Work out the finished part from the listing and answer in its coordinate system (mm). A direction names the side the tool comes from. Give positions to 0.01 mm unless a question says otherwise; leave off trailing zeros. Write each loop counter-clockwise with the first axis right and the second up, starting at its lowest first coordinate (ties: lowest second). Pieces come first, ordered by that corner, then holes.
1) Determine the mould class of faces 1 (the face through (20, 20, -8)), 2 (the face through (-28.977, 29.58, -1.162)), 3 (the face through (3.228, 51.208, -0.406)), 4 (the face through (20, 20, 8)) for opening direction Z: pulls with the +Z half, pulls with the -Z half, needs draft (parallel to the pull), parting line crosses it, or undercut.
2) Find section C-C (x = -15). Determine the outline of the cut face in (y, z).
3) Find section A-A (z = 0). Determine the outline of the cut face in (x, y).
4) Find section B-B (y = 41.5). Determine the outline of the cut face in (x, z), plus the area to 3 significant figures.
5) Given pin 1 Ø2 at (x, y) = (-17.5, 9.5) entering from +Z; pin 2 Ø14 at (x, y) = (21, 17) entering from -Z; pin 3 Ø13 at (y, z) = (26.5, -4) entering from +X, each flat-ended and moving along its own axis, determine where each tip first touches the part or whether it passes through.
6) A tool of negligible diameter and unlimited length cuts with its end or side. For faces 5 (the face through (15.144, 22, 0)), 6 (the face through (-1, 0, 0)), from which of +Z, -Z, +X, -X, +Y, -Y can it reach the whole face along a straight path? Write none if from no direction.
7) Find section D-D (z = -14.5). Determine the outline of the cut face in (x, y).
8) Straight lines are drawn through the part: probe 1 along Z at (x, y) = (25.5, 11); probe 2 along X at (y, z) = (3, 0); probe 3 along Z at (x, y) = (23.5, 19.5). For each, find the intervals that lie inside material, in ascending order.
```python
from build123d import *

# Parameters (mm, degrees)
SKETCH1_R               = 29
BOSS_EXTRUDE1_DEPTH     = 60
CUT_EXTRUDE1_DEPTH      = 30
CUT_EXTRUDE1_DEPTH_BACK = 30
CUT_EXTRUDE2_DEPTH      = 70.969655115


with BuildPart() as part:
    # Sketch1 → Boss-Extrude1 (new body)
    with BuildSketch(Plane(origin=(0, 0, 0), x_dir=(1, 0, 0), z_dir=(0, 1, 0))):
        Circle(SKETCH1_R)
    extrude(amount=BOSS_EXTRUDE1_DEPTH)

    # Sketch2 → Cut-Extrude1 (cut, two sides)
    with BuildSketch(Plane.XY) as cut_extrude1_sk:
        Polygon((-12, 60), (29, 36.328638963), (29, 60), align=None)
    extrude(amount=CUT_EXTRUDE1_DEPTH, mode=Mode.SUBTRACT)
    extrude(cut_extrude1_sk.sketch, amount=-CUT_EXTRUDE1_DEPTH_BACK, mode=Mode.SUBTRACT)

    # Sketch7 → Cut-Extrude2 (cut, through all, along a direction that is not the sketch's normal)
    with BuildSketch(Plane(origin=(22.980762114, 39.803847577, 0), x_dir=(0.866025404, -0.5, 0), z_dir=(0.5, 0.866025404, 0))):
        with BuildLine():
            Line((5.651055494, 8), (-9.049582772, 8))
            Line((-9.049582772, 8), (-9.049582772, -8))
            Line((-9.049582772, -8), (5.651055494, -8))
            ThreePointArc((5.651055494, -8), (6.950417228, 0), (5.651055494, 8))
        make_face()
    extrude(amount=-CUT_EXTRUDE2_DEPTH, dir=(0, 1, 0), mode=Mode.SUBTRACT)


solid = part.part
```
Results:
1. face 1: undercut
1. face 2: parting line crosses it
1. face 3: needs draft
1. face 4: undercut
2. outline: (0, -24.82) - (60, -24.82) - (60, 24.82) - (0, 24.82) - close
3. outline: (-29, 0) - (15.14, 0) - (15.14, 44.33) - (-12, 60) - (-29, 60) - close
4. outline: (15.14, -8) - (15.14, 8) - (20.04, 8) - (20.04, 20.96) arc R29 ccw (long way) to (20.04, -20.96) - (20.04, -8) - close
4. area: 2,300 mm2
5. pin 1: stops at z = 23.85
5. pin 2: stops at z = -25.4
5. pin 3: stops at x = 27.87
6. face 5: +X, +Y, -Y
6. face 6: +Z, -Z, +X, -X, -Y
7. outline: (-25.11, 0) - (25.11, 0) - (25.11, 38.57) - (-12, 60) - (-25.11, 60) - close
8. probe 1: z = -13.81 to -8, 8 to 13.81
8. probe 2: x = -29 to 15.14
8. probe 3: z = -16.99 to -8, 8 to 16.99
